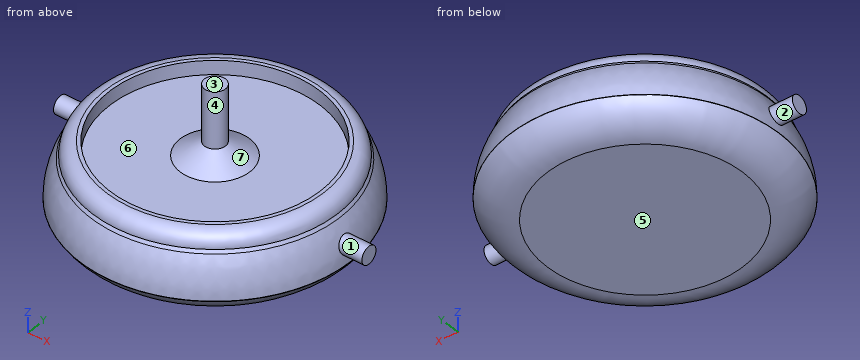
```python
from build123d import *

# Parameters (mm, degrees)
SKETCH1_R                = 15
BOSS_EXTRUDE1_DEPTH      = 80
SKETCH2_R                = 15
BOSS_EXTRUDE2_DEPTH      = 20
BOSS_EXTRUDE2_DRAFT      = -60
SKETCH3_R                = 175
BOSS_EXTRUDE5_DEPTH      = 30
BOSS_EXTRUDE5_DRAFT      = -30
SKETCH6_R                = 175
SKETCH6_R_2              = 150
BOSS_EXTRUDE6_DEPTH      = 20
SKETCH7_R                = 192.320508076
BOSS_EXTRUDE7_DEPTH      = 30
SKETCH9_R                = 192.320508076
BOSS_EXTRUDE8_DEPTH      = 30
BOSS_EXTRUDE8_TAPER      = 30
FILLET2_R                = 60
FILLET3_R                = 110
FILLET4_R                = 20
BOSS_EXTRUDE9_DEPTH      = 30
BOSS_EXTRUDE9_DEPTH_BACK = 414
SKETCH10_R               = 12.5


with BuildPart() as part:
    # Sketch1 → Boss-Extrude1 (new body)
    with BuildSketch(Plane.XY):
        Circle(SKETCH1_R)
    extrude(amount=BOSS_EXTRUDE1_DEPTH)


with BuildPart() as boss_extrude2_tool:
    # Sketch2 → Boss-Extrude2 (with draft: the straight prism first)
    with BuildSketch(Plane(origin=(0, 0, 0), x_dir=(-1, 0, 0), z_dir=(0, 0, -1))):
        Circle(SKETCH2_R)
    extrude(amount=BOSS_EXTRUDE2_DEPTH)
    # Boss-Extrude2: the draft: its side faces are tilted about the plane it starts from
    boss_extrude2_sides = [boss_extrude2_tool.faces().sort_by_distance(p)[0] for p in [
        (15, 0, -10),
    ]]
    draft(boss_extrude2_sides, Plane(origin=(0, 0, 0), x_dir=(-1, 0, 0), z_dir=(0, 0, -1)), BOSS_EXTRUDE2_DRAFT)


with BuildPart() as part_1:
    add(part.part)

    # Boss-Extrude2: add boss_extrude2_tool
    add(boss_extrude2_tool.part)


with BuildPart() as boss_extrude5_tool:
    # Sketch3 → Boss-Extrude5 (with draft: the straight prism first)
    with BuildSketch(Plane(origin=(0, 0, -20), x_dir=(-1, 0, 0), z_dir=(0, 0, -1))):
        Circle(SKETCH3_R)
    extrude(amount=BOSS_EXTRUDE5_DEPTH)
    # Boss-Extrude5: the draft: its side faces are tilted about the plane it starts from
    boss_extrude5_sides = [boss_extrude5_tool.faces().sort_by_distance(p)[0] for p in [
        (175, 0, -35),
    ]]
    draft(boss_extrude5_sides, Plane(origin=(0, 0, -20), x_dir=(-1, 0, 0), z_dir=(0, 0, -1)), BOSS_EXTRUDE5_DRAFT)


with BuildPart() as part_2:
    add(part_1.part)

    # Boss-Extrude5: add boss_extrude5_tool
    add(boss_extrude5_tool.part)

    # Sketch6 → Boss-Extrude6 (add)
    with BuildSketch(Plane.XY.offset(-20)):
        Circle(SKETCH6_R)
        Circle(SKETCH6_R_2, mode=Mode.SUBTRACT)
    extrude(amount=BOSS_EXTRUDE6_DEPTH)

    # Sketch7 → Boss-Extrude7 (add)
    with BuildSketch(Plane(origin=(0, 0, -50), x_dir=(-1, 0, 0), z_dir=(0, 0, -1))):
        Circle(SKETCH7_R)
    extrude(amount=BOSS_EXTRUDE7_DEPTH)

    # Sketch9 → Boss-Extrude8 (add)
    with BuildSketch(Plane(origin=(0, 0, -80), x_dir=(-1, 0, 0), z_dir=(0, 0, -1))):
        Circle(SKETCH9_R)
    extrude(amount=BOSS_EXTRUDE8_DEPTH, taper=BOSS_EXTRUDE8_TAPER)

    # Fillet2
    fillet2_edges = [part_2.edges().sort_by_distance(p)[0] for p in [
        (175, 0, -110),
    ]]
    fillet(fillet2_edges, radius=FILLET2_R - 0.0001)  # a hair under: the kernel refuses the full size

    # Fillet3
    fillet3_edges = [part_2.edges().sort_by_distance(p)[0] for p in [
        (192.320508076, 0, -50),
    ]]
    fillet(fillet3_edges, radius=FILLET3_R)

    # Fillet4
    fillet4_edges = [part_2.edges().sort_by_distance(p)[0] for p in [
        (-175, 0, 0),
    ]]
    fillet(fillet4_edges, radius=FILLET4_R - 0.0001)  # a hair under: the kernel refuses the full size

    # Sketch10 → Boss-Extrude9 (add, two sides: drawn at the far end of the back side and taken through both)
    with BuildSketch(Plane.ZY.offset(192.320508076).offset(-BOSS_EXTRUDE9_DEPTH_BACK)):
        with Locations((-54.474411167, 0)):
            Circle(SKETCH10_R)
    extrude(amount=BOSS_EXTRUDE9_DEPTH + BOSS_EXTRUDE9_DEPTH_BACK)


solid = part_2.part
```
Read the model definition and answer for the solid it produces. Units are mm, in the model's axes. Face numbers are marked on the shaded views. A direction names the side the tool comes from. Coordinates: 2 decimals unless noted, no trailing zeros. Order: outer loops, then holes, each group sorted by start corner. A loop starts at its lowest first (then second) coordinate and runs counter-clockwise, first axis right, second up. Notation, with made-up numbers: (72, -30) - (130, -30) arc R18 cw to (130, -12) - close; hole circle Ø8 at (88, 10). An arc over 180 degrees is marked (long way). Answer as a JSON object with one key per item and string values. Group by question number.
Item 1: Flat-ended cylindrical pins translate along their axes: P1, Ø5, axis at y = 44.5, z = -8, coming from the +X side; P2, Ø2, axis at x = 49, z = -15.5, coming from the -Y side; P3, Ø3, axis at y = 104.5, z = -90.5, coming from the -X side. Find the tip coordinate at first contact, or state that the pin passes through.
Item 2: Consider probe 1 along Y at (x, z) = (0, -12); probe 2 along Y at (x, z) = (0, -14); probe 3 along X at (y, z) = (-8, -12). Determine where each line is inside the solid, lowest interval first. Write a range as from..to.
Item 3: Section A-A (z = -9.5) is taken. Give the vertices of the cut face in (x, y).
Item 4: A tool of negligible diameter and unlimited length cuts with its end or side. For the marked faces 1, 2 and 3, from which of +Z, -Z, +X, -X, +Y, -Y can it reach the whole face along a straight path? Write none if from no direction.
Item 5: The mould has two halves that part along X. Classify the marked faces 4, 5, 6 and 7: +X half, -X half, draft (parallel to the pull), parting line (faces both ways), or undercut.
Results are:
{
 "1": {"P1": "stops at x = 166.91", "P2": "stops at y = -167.83", "P3": "stops at x = -154.12"},
 "2": {"probe 1": "y = -173.33..-150, -35.78..35.78, 150..173.33", "probe 2": "y = -174.08..-150, -39.25..39.25, 150..174.08", "probe 3": "x = -173.15..-149.79, -34.88..34.88, 149.79..173.15"},
 "3": {"outline": "circle Ø344.04 at (0, 0); circle Ø62.91 at (0, 0); hole circle Ø300 at (0, 0)"},
 "4": {"face 1": "+X", "face 2": "-X", "face 3": "+Z, +X, -X, +Y, -Y"},
 "5": {"face 4": "parting line", "face 5": "draft", "face 6": "undercut", "face 7": "undercut"}
}
